from build123d import *

# Parameters (mm, degrees)
FILLET_1_R               = 2
SKETCH_2_R               = 4
CUT_EXTRUDE_1_DEPTH      = 20
CUT_EXTRUDE_2_DEPTH      = 43.866070499
CUT_EXTRUDE_2_DEPTH_BACK = 43.866070499
SKETCH_3_R               = 1.5
CHAMFER_1_SIZE           = 0.5
CUT_EXTRUDE_3_DEPTH      = 43.866070499
CUT_EXTRUDE_3_DEPTH_BACK = 43.866070499
SKETCH_4_OUTSIDE_W       = 49.124
SKETCH_4_OUTSIDE_H       = 49.124


with BuildPart() as part:
    # 草图1 → 旋转1 (revolve)
    with BuildSketch(Plane.XY, mode=Mode.PRIVATE) as revolve_1_sk:
        with BuildLine():
            Line((0, 0), (9, 0))
            Line((9, 0), (9, 3))
            Line((9, 3), (7.5, 3))
            Line((7.5, 3), (7.5, 12))
            ThreePointArc((7.5, 12), (9.843145751, 17.656854249), (15.5, 20))
            Line((15.5, 20), (17.5, 20))
            Line((17.5, 20), (17.5, 30.310889132))
            ThreePointArc((17.5, 30.310889132), (9.058666579, 33.80740392), (0, 35))
            Line((0, 35), (0, 0))
        make_face()
    revolve(revolve_1_sk.sketch.rotate(Axis((0, 0, 0), (0, 1, 0)), 90), axis=Axis((0, 0, 0), (0, 1, 0)))

    # 圆角1
    # the kernel refuses this fillet: 2 mm, written as the material it adds along each edge
    with BuildSketch(Plane(origin=(0, 3, 0), x_dir=(0, 0, -1), z_dir=(1, 0, 0))) as fillet_1_piece_1:
        with BuildLine():
            CenterArc((9.5, 1.936491673), FILLET_1_R, 180, 75.522487814)
            Line((7.5, 1.936491673), (7.46, 1.936491673))
            Line((7.46, 1.936491673), (7.46, 0))
            Line((7.46, 0), (7.5, -0.04))
            ThreePointArc((7.5, -0.04), (8.25, -0.04), (8.99, -0.038729833))
            Line((8.99, -0.038729833), (9, 0))
        make_face()
    revolve(axis=Axis((0, 3, 0), (0, 1, 0)))

    # 草图2 → 切除-拉伸1 (cut)
    with BuildSketch(Plane.XZ):
        with Locations(Location((0, 0, 0), (0, 0, 270))):
            Circle(SKETCH_2_R)
    extrude(amount=-CUT_EXTRUDE_1_DEPTH, mode=Mode.SUBTRACT)

    # 草图3 → 切除-拉伸2 (cut, two sides: drawn at the far end of the back side and taken through both)
    with BuildSketch(Plane.XY.offset(-CUT_EXTRUDE_2_DEPTH_BACK)):
        with Locations((0, 8)):
            Circle(SKETCH_3_R)
    extrude(amount=CUT_EXTRUDE_2_DEPTH + CUT_EXTRUDE_2_DEPTH_BACK, mode=Mode.SUBTRACT)

    # 倒角1
    chamfer_1_edges = [part.edges().sort_by_distance(p)[0] for p in [
        (0, 0, 4),
    ]]
    chamfer(chamfer_1_edges, length=CHAMFER_1_SIZE)

    # 草图4 outside → 切除-拉伸3 (cut, two sides: drawn at the far end of the back side and taken through both)
    with BuildSketch(Plane(origin=(0, 0, 0), x_dir=(1, 0, 0), z_dir=(0, 1, 0)).offset(-CUT_EXTRUDE_3_DEPTH_BACK)):
        Rectangle(SKETCH_4_OUTSIDE_W, SKETCH_4_OUTSIDE_H)
        with BuildLine():
            ThreePointArc((2.625011684, -16.442929558), (0, -16), (-2.625011684, -16.442929558))
            ThreePointArc((-2.625011684, -16.442929558), (-5.975744703, -16.418223636), (-8.558435773, -14.283339803))
            ThreePointArc((-8.558435773, -14.283339803), (-10.284601755, -12.25671109), (-12.580187001, -10.908689831))
            ThreePointArc((-12.580187001, -10.908689831), (-15.13111675, -8.735954329), (-15.737296016, -5.440416612))
            ThreePointArc((-15.737296016, -5.440416612), (-15.756924048, -2.778370843), (-16.648953007, -0.270152895))
            ThreePointArc((-16.648953007, -0.270152895), (-17.206471106, 3.033965099), (-15.552500552, 5.948137976))
            ThreePointArc((-15.552500552, 5.948137976), (-13.856406461, 8), (-12.927488868, 10.494791583))
            ThreePointArc((-12.927488868, 10.494791583), (-11.230726403, 13.384258538), (-8.090517233, 14.553492698))
            ThreePointArc((-8.090517233, 14.553492698), (-5.472322293, 15.035081933), (-3.157109015, 16.349106443))
            ThreePointArc((-3.157109015, 16.349106443), (0, 17.471908657), (3.157109015, 16.349106443))
            ThreePointArc((3.157109015, 16.349106443), (5.472322293, 15.035081933), (8.090517233, 14.553492698))
            ThreePointArc((8.090517233, 14.553492698), (11.230726403, 13.384258538), (12.927488868, 10.494791583))
            ThreePointArc((12.927488868, 10.494791583), (13.856406461, 8), (15.552500552, 5.948137976))
            ThreePointArc((15.552500552, 5.948137976), (17.206471106, 3.033965099), (16.648953007, -0.270152895))
            ThreePointArc((16.648953007, -0.270152895), (15.756924048, -2.778370843), (15.737296016, -5.440416612))
            ThreePointArc((15.737296016, -5.440416612), (15.13111675, -8.735954329), (12.580187001, -10.908689831))
            ThreePointArc((12.580187001, -10.908689831), (10.284601755, -12.25671109), (8.558435773, -14.283339803))
            ThreePointArc((8.558435773, -14.283339803), (5.975744703, -16.418223636), (2.625011684, -16.442929558))
        make_face(mode=Mode.SUBTRACT)
    extrude(amount=CUT_EXTRUDE_3_DEPTH + CUT_EXTRUDE_3_DEPTH_BACK, mode=Mode.SUBTRACT)


solid = part.part
Geometry: final body of the model. Coordinates: model frame, mm. A direction names the side the tool comes from. Round coordinates to 2 decimals unless told otherwise and drop trailing zeros. Order: outer loops, then holes, each group sorted by start corner. A loop starts at its lowest first (then second) coordinate and runs counter-clockwise, first axis right, second up. Notation, with made-up numbers: (13, 36) -> (58, 36) arc R10 ccw to (58, 42) -> close; hole circle Ø3 at (-32, -29.75). An arc over 180 degrees is marked (long way). Put each result on its own line as item: value. Start each with the question number.
Q1. Section A-A on x = 0. Return the cut outline in (y, z), and give its area (3 significant figures).
Q2. Section D-D on y = 19. Return the cut outline in (x, z), and give its area (3 significant figures).
Q3. Section C-C on y = 26.5. Return the cut outline in (x, z).
Q4. First-contact query: pin 1 (5 mm diameter, centred on x = 0, y = 8, fed in from -Z); pin 2 (10 mm diameter, centred on y = 24, z = -7.5, fed in from +X); pin 3 (9 mm diameter, centred on x = -1, z = 0, fed in from -Y); pin 4 (3 mm diameter, centred on x = -5, y = 9.5, fed in from -Z). Flat tips, straight axial feed; report the tip coordinate or a pass-through.
Q5. Line query: probe 1 along X at (y, z) = (9.5, 0); probe 2 along Y at (x, z) = (0, 5); probe 3 along X at (y, z) = (11, -2). Output: solid intervals per line, ascending.
Q6. Reachability of faces 4 (the cylindrical face through (13.84, 25.49, -8.03)), 5 (the flat face through (0, 20, 0)) from +Z, -Z, +X, -X, +Y, -Y: full face, straight path, thin tool, end or side. Return the list, or none.
Q7. Section B-B on y = 8. Return the cut outline in (x, z), and give its area (3 significant figures).
Q8. Pull-direction query (X, two-part tool) for faces 1 (the cylindrical face through (-17.215, 25.317, -2.987)), 2 (the cylindrical face through (15.155, 25.317, 8.694)), 3 (the cylindrical face through (1.386, 7.425, -5.631)); classes: +X half, -X half, draft (parallel to the pull), parting line (faces both ways), or undercut.
Ans:
1. outline: (0, -9) -> (3, -9) arc R2 cw to (4.94, -7.5) -> (6.5, -7.5) -> (6.5, -4) -> (0.5, -4) -> (0, -4.5) -> close; (0, 4.5) -> (0.5, 4) -> (6.5, 4) -> (6.5, 7.5) -> (4.94, 7.5) arc R2 cw to (3, 9) -> (0, 9) -> close; (9.5, -7.5) -> (12, -7.5) arc R8 cw to (20, -15.5) -> (20, -17.47) -> (30.33, -17.47) arc R35 ccw to (31.13, 16) -> (20, 16) -> (20, 15.5) arc R8 cw to (12, 7.5) -> (9.5, 7.5) -> (9.5, 4) -> (20, 4) -> (20, -4) -> (9.5, -4) -> close
1. area: 612 mm2
2. outline: circle Ø23.25 at (0, 0); hole circle Ø8 at (0, 0)
2. area: 374 mm2
3. outline: (-16.65, 0.27) arc R5 ccw to (-15.55, -5.95) arc R8 cw to (-12.93, -10.49) arc R5 ccw to (-8.09, -14.55) arc R8 cw to (-3.16, -16.35) arc R5 ccw to (3.16, -16.35) arc R8 cw to (8.09, -14.55) arc R5 ccw to (12.93, -10.49) arc R8 cw to (15.55, -5.95) arc R5 ccw to (16.65, 0.27) arc R8 cw to (15.74, 5.44) arc R5 ccw to (12.58, 10.91) arc R8 cw to (8.56, 14.28) arc R5 ccw to (2.63, 16.44) arc R8 cw to (-2.63, 16.44) arc R5 ccw to (-8.56, 14.28) arc R8 cw to (-12.58, 10.91) arc R5 ccw to (-15.74, 5.44) arc R8 cw to start
4. pin 1: stops at z = -7.5
4. pin 2: stops at x = 17.27
4. pin 3: stops at y = 0
4. pin 4: stops at z = -6.63
5. probe 1: x = -7.5 to -4, 4 to 7.5
5. probe 2: y = 0 to 6.5, 9.5 to 34.64
5. probe 3: x = -7.23 to -3.46, 3.46 to 7.23
6. face 4: -Z, +X, +Y, -Y
6. face 5: -Y
7. outline: (-1.5, -7.35) -> (-1.5, -3.71) arc R4 cw to (-1.5, 3.71) -> (-1.5, 7.35) arc R7.5 ccw to start; (1.5, -7.35) arc R7.5 ccw to (1.5, 7.35) -> (1.5, 3.71) arc R4 cw to (1.5, -3.71) -> close
7. area: 105 mm2
8. face 1: -X half
8. face 2: +X half
8. face 3: undercut
